Verification items for the finished model (mm, model axes). Face numbers are marked on the shaded views. Coordinates: 2 decimals unless noted, no trailing zeros. Order: outer loops, then holes, each group sorted by start corner. A loop starts at its lowest first (then second) coordinate and runs counter-clockwise, first axis right, second up. Notation, with made-up numbers: (86, -30.5) -> (109, -30.5) arc R36 ccw to (109, 3.5) -> close; hole circle Ø9 at (-2.75, 60). An arc over 180 degrees is marked (long way). Use CSV: the item, a comma, the result in double quotes. Start each with the question number.
1) Sectioned sample at B-B on y = 15.5. Record the boundary of the cut face in (x, z), then the cut area to 3 significant figures.
2) Sectioned sample at A-A on y = 23. Record the boundary of the cut face in (x, z).
3) Go/stop test with flat-tipped pins: pin 1 (12 mm diameter, centred on x = -24.5, y = 4, fed in from +Z); pin 2 (1.2 mm diameter, centred on y = 16.5, z = -17, fed in from +X); pin 3 (12 mm diameter, centred on x = 17.5, y = 7.5, fed in from -Z). Record where each tip stops, or that it passes through.
4) Scan lines: line 1 along Y through (x, z) = (37.85, 0); line 2 along Z through (x, y) = (-1, 12.5); line 3 along Y through (x, z) = (0, -16.15). Record each from-to range of solid material in increasing order.
5) Sectioned sample at C-C on x = 0. Give the number of separate pieces and of enclosed holes in the cut face, then the cut area to 4 significant figures.
6) Release check for a two-part mould opening along X. For the marked faces 1 and 2 record: released by +X, released by -X, zero draft, split by the parting line, or undercut.
7) Sectioned sample at D-D on z = -4. Record the boundary of the cut face in (x, y).
from build123d import *

# Parameters (mm, degrees)
CROQUIS2_R                 = 38.79
SALIENTE_EXTRUIR1_DEPTH    = 5
CROQUIS4_W                 = 6
CROQUIS4_H                 = 25
SALIENTE_EXTRUIR3_DEPTH    = 2.5
CORTAR_EXTRUIR1_DEPTH      = 73.788929103
CORTAR_EXTRUIR1_DEPTH_BACK = 73.788929103
CROQUIS5_R                 = 1.25
REDONDEO1_R                = 5
CORTAR_EXTRUIR2_START      = 50
CROQUIS6_R                 = 2
CORTAR_EXTRUIR2_DEPTH      = 17
MATRIZC1_COUNT             = 4


with BuildPart() as part:
    # Croquis2 → Saliente-Extruir1 (new body)
    with BuildSketch(Plane(origin=(0, 0, 0), x_dir=(1, 0, 0), z_dir=(0, 1, 0))):
        with Locations(Location((0, 0, 0), (0, 0, 270))):
            Circle(CROQUIS2_R)
        with BuildLine():
            Line((-12.586494468, 15), (12.586494468, 15))
            Line((12.586494468, 15), (23.64815616, 28.182775062))
            ThreePointArc((23.64815616, 28.182775062), (36.79, 0), (23.64815616, -28.182775062))
            Line((23.64815616, -28.182775062), (12.586494468, -15))
            Line((12.586494468, -15), (-12.586494468, -15))
            Line((-12.586494468, -15), (-23.64815616, -28.182775062))
            ThreePointArc((-23.64815616, -28.182775062), (-36.79, 0), (-23.64815616, 28.182775062))
            Line((-23.64815616, 28.182775062), (-12.586494468, 15))
        make_face(mode=Mode.SUBTRACT)
        with BuildLine():
            Line((-11.420725322, 17.5), (-21.678382494, 29.724599786))
            ThreePointArc((-21.678382494, 29.724599786), (0, 36.79), (21.678382494, 29.724599786))
            Line((21.678382494, 29.724599786), (11.420725322, 17.5))
            Line((11.420725322, 17.5), (-11.420725322, 17.5))
        make_face(mode=Mode.SUBTRACT)
        with BuildLine():
            ThreePointArc((21.678382494, -29.724599786), (0, -36.79), (-21.678382494, -29.724599786))
            Line((-21.678382494, -29.724599786), (-11.420725322, -17.5))
            Line((-11.420725322, -17.5), (11.420725322, -17.5))
            Line((11.420725322, -17.5), (21.678382494, -29.724599786))
        make_face(mode=Mode.SUBTRACT)
    extrude(amount=SALIENTE_EXTRUIR1_DEPTH)

    # Croquis4 → Saliente-Extruir3 (add)
    with BuildSketch(Plane.XY.offset(15)):
        with Locations((0, 12.5)):
            Rectangle(CROQUIS4_W, CROQUIS4_H)
    saliente_extruir3 = extrude(amount=SALIENTE_EXTRUIR3_DEPTH)

    # Simetría1: Saliente-Extruir3 across plane
    add(saliente_extruir3.mirror(Plane.XY))

    # Croquis5 → Cortar-Extruir1 (cut, two sides: drawn at the far end of the back side and taken through both)
    with BuildSketch(Plane(origin=(0, 0, -17.5), x_dir=(-1, 0, 0), z_dir=(0, 0, -1)).offset(-CORTAR_EXTRUIR1_DEPTH_BACK)):
        with Locations(Location((0, 23, 0), (0, 0, 180))):
            Circle(CROQUIS5_R)
    extrude(amount=CORTAR_EXTRUIR1_DEPTH + CORTAR_EXTRUIR1_DEPTH_BACK, mode=Mode.SUBTRACT)

    # Redondeo1
    redondeo1_edges = [part.edges().sort_by_distance(p)[0] for p in [
        (-11.420725322, 2.5, -17.5),
        (11.420725322, 2.5, -17.5),
        (11.420725322, 2.5, 17.5),
        (-11.420725322, 2.5, 17.5),
    ]]
    fillet(redondeo1_edges, radius=REDONDEO1_R)

    # Croquis6 → Cortar-Extruir2 (cut)
    with BuildSketch(Plane.XY.offset(CORTAR_EXTRUIR2_START)):
        with Locations((0, 2.5)):
            Circle(CROQUIS6_R)
    cortar_extruir2 = extrude(amount=-CORTAR_EXTRUIR2_DEPTH, mode=Mode.SUBTRACT)

    # MatrizC1: Cortar-Extruir2 ×4 about axis
    matrizc1_axis = Axis((0, 0, 0), (0, -1, 0))
    for i in range(1, MATRIZC1_COUNT):
        add(cortar_extruir2.rotate(matrizc1_axis, i * 360 / MATRIZC1_COUNT), mode=Mode.SUBTRACT)


solid = part.part
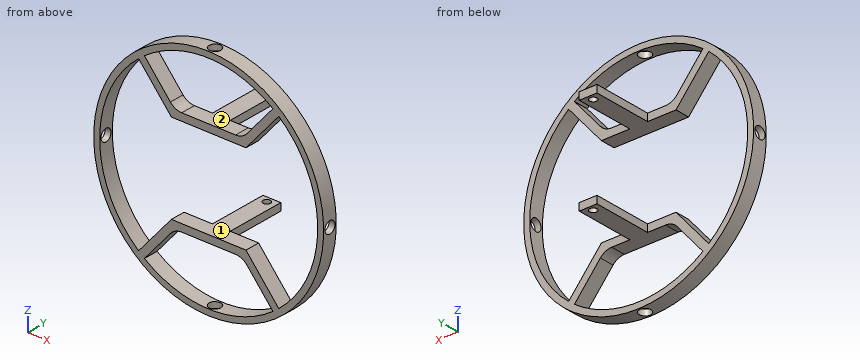
Answers follow:
1,outline,"(-3, -17.5) -> (3, -17.5) -> (3, -15) -> (-3, -15) -> close; (-3, 15) -> (3, 15) -> (3, 17.5) -> (-3, 17.5) -> close"
1,area,"30.0 mm²"
2,outline,"(-3, -17.5) -> (-1.25, -17.5) -> (-1.25, -15) -> (-3, -15) -> close; (-3, 15) -> (-1.25, 15) -> (-1.25, 17.5) -> (-3, 17.5) -> close; (1.25, -17.5) -> (3, -17.5) -> (3, -15) -> (1.25, -15) -> close; (1.25, 15) -> (3, 15) -> (3, 17.5) -> (1.25, 17.5) -> close"
3,pin 1,"stops at z = 34.09"
3,pin 2,"stops at x = 3"
3,pin 3,"stops at z = -36.87"
4,line 1,"y = 0 to 0.5, 4.5 to 5"
4,line 2,"z = -17.5 to -15, 15 to 17.5"
4,line 3,"y = 0 to 21.75, 24.25 to 25"
5,separate pieces,"8"
5,enclosed holes,"0"
5,area,"116.5 mm²"
6,face 1,"undercut"
6,face 2,"undercut"
7,outline,"(-38.58, 0) -> (-36.57, 0) -> (-36.57, 5) -> (-38.58, 5) -> close; (36.57, 0) -> (38.58, 0) -> (38.58, 5) -> (36.57, 5) -> close"
